Autodesk Inventor part; units mm, degrees
ref_plane "YZ Plane" through (0, 0, 0) normal (1, 0, 0) x (0, 1, 0)
ref_plane "XZ Plane" through (0, 0, 0) normal (0, 1, 0) x (-1, 0, 0)
ref_plane "XY Plane" through (0, 0, 0) normal (0, 0, 1) x (1, 0, 0)
sketch "スケッチ1" plane through (0, 0, 0) normal (1, 0, 0) x (0, 1, 0)
  circle A0 centre (0, 0) radius 4.575
  circle A1 centre (0, 0) radius 3.575
  line L0 (0, 0) -> (0, 6)
  line L1 (0, 6) -> (0, -6)
  line L2 (0, 0) -> (11.5, 0)
  line L3 (11.5, 0) -> (11.5, 9.5)
  line L4 (11.5, 9.5) -> (11.5, -9.5)
  circle A2 centre (11.5, 9.5) radius 1.65
  circle A3 centre (11.5, -9.5) radius 1.65
  line L5 (0, 0) -> (0, 11.25)
  line L6 (0, 11.25) -> (0, -11.25)
  line L7 (-2.5, -11.25) -> (2.5, -11.25)
  line L8 (2.5, -11.25) -> (2.5, 11.25)
  line L9 (2.5, 11.25) -> (-2.5, 11.25)
  line L10 (-2.5, 11.25) -> (-2.5, -11.25)
  line L11 (-2.5, -11.25) -> (2.5, 11.25) construction
  line L12 (2.5, -11.25) -> (-2.5, 11.25) construction
  circle A4 centre (11.5, 9.5) radius 2.5
  circle A5 centre (11.5, -9.5) radius 2.5
  line L13 (2.5, 11.25) -> (11.2899, 11.9912)
  line L14 (2.5, -11.25) -> (11.2899, -11.9912)
  line L15 (14, 9.5) -> (14, -9.5)
  line L16 (0, -3.575) -> (14, -3.575)
  line L17 (0, 3.575) -> (14, 3.575)
  circle A6 centre (0, 0) radius 6
  line L18 (0, 0) -> (0, 6.15)
  line L19 (0, 6.15) -> (0, -6.15)
  circle A7 centre (0, 6.15) radius 1.25
  circle A8 centre (0, -6.15) radius 1.25
  point P0 (0, 4.575)
  point P1 (0, -4.575)
  point P2 (2.5, 3.575)
  point P3 (2.5, 2.5555)
  point P4 (2.5, -2.5555)
  point P5 (2.5, -3.575)
  point P6 (0, 7.4)
  point P7 (0, 4.9)
  point P8 (0, -4.9)
  point P9 (0, -7.4)
  point P10 (2.5, 5.4544)
  point P11 (2.5, -5.4544)
  point P12 (4.8186, 3.575)
  point P13 (4.8186, -3.575)
  point P14 (2.8548, 3.575)
  point P15 (2.8548, -3.575)
  dimension "d0" = 9.15
  dimension "d1" = 7.15
  dimension "d2" = 6
  dimension "d3" = 12
  dimension "d6" = 11.5
  dimension "d7" = 9.5
  dimension "d8" = 19
  dimension "d9" = 3.3
  dimension "d10" = 3.3
  dimension "d11" = 11.25
  dimension "d12" = 22.5
  dimension "d13" = 5
  dimension "d14" = 5
  dimension "d15" = 5
  dimension "d28" = 12
  dimension "d29" = 6.15
  dimension "d30" = 12.3
  dimension "d31" = 2.5
  dimension "d32" = 2.5
extrude "押し出し7" add sketch "スケッチ1" along normal blind 2 contours L2 A6 L16 A0 | A0 L17 A6 L2 | A0 L8 A6 L17 | L16 A6 L8 A0 | A6 L17 L3 L2 | L2 L4 L16 A6 | A0 L0 A7 A6 L8 | A6 L8 L13 A4 L3 L17 | L8 A6 A8 L1 A0 | L16 L4 A5 L14 L8 A6 | L3 L17 L15 L16 L4 | A6 A7 L5 L9 L8 | L3 A4 L15 L17 | L8 L7 L6 A8 A6 | L16 L15 A5 L4 | A4 | A5
extrude "押し出し8" add sketch "スケッチ1" along normal blind 10 contours L2 A6 L16 A0 | A0 L17 A6 L2 | A0 L8 A6 L17 | L16 A6 L8 A0 | A6 L17 L3 L2 | L2 L4 L16 A6 | A0 L0 A7 A6 L8 | L8 A6 A8 L1 A0 | L3 L17 L15 L16 L4 | A6 A7 L5 L9 L8 | L8 L7 L6 A8 A6 | L0 A6 A7 | A6 L5 A7 | A8 A6 L1 | A8 L6 A6 picked at (0.2292, 5.6392) picked at (0.3961, 6.4211) picked at (0.2292, -5.6392) picked at (0.3961, -6.4211)
sketch "スケッチ6" plane through (10, 0, 0) normal (1, 0, 0) x (0, 0, -1)
  line L0 (0, 0) -> (-6.15, 0)
  line L1 (-6.15, 0) -> (6.15, 0)
  circle A0 centre (-6.15, 0) radius 1.25
  circle A1 centre (6.15, 0) radius 1.25
  line L2 (-11.25, 2.5) -> (11.25, 2.5)
  line L3 (11.25, 2.5) -> (11.25, -2.5)
  line L4 (11.25, -2.5) -> (-11.25, -2.5)
  line L5 (-11.25, -2.5) -> (-11.25, 2.5)
  line L6 (-11.25, 2.5) -> (11.25, -2.5) construction
  line L7 (11.25, 2.5) -> (-11.25, -2.5) construction
  line L8 (0, 0) -> (0, 11.5)
  line L9 (0, 11.5) -> (-9.5, 11.5)
  line L10 (-9.5, 11.5) -> (9.5, 11.5)
  circle A2 centre (-9.5, 11.5) radius 1.65
  circle A3 centre (-9.5, 11.5) radius 2.5
  circle A4 centre (9.5, 11.5) radius 1.65
  circle A5 centre (9.5, 11.5) radius 2.5
  circle A6 centre (0, 0) radius 6
  circle A7 centre (0, 0) radius 4.575
  arc A8 (11.9912, 11.2899) -> (9.5, 14) centre (9.5, 11.5) ccw
  line L11 (11.25, 2.5) -> (11.9912, 11.2899)
  line L12 (-11.9912, 11.2899) -> (-11.25, 2.5)
  line L13 (-11.25, 2.5) -> (-11.9912, 11.2899)
  line L14 (9.5, 14) -> (-9.5, 14)
  arc A9 (-9.5, 14) -> (-11.9912, 11.2899) centre (-9.5, 11.5) ccw
  line L15 (-9.5, 14) -> (9.5, 14)
  circle A10 centre (0, 0) radius 3.575
  line L16 (-3.575, 14) -> (-3.575, 4.8186)
  line L17 (3.575, -14) -> (-3.575, -14)
  line L18 (-3.575, -14) -> (-3.575, 14)
  line L19 (-3.575, 14) -> (3.575, 14)
  line L20 (3.575, 14) -> (3.575, -14)
  line L21 (3.575, -14) -> (-3.575, 14) construction
  line L22 (-3.575, -14) -> (3.575, 14) construction
  point P0 (-5.4544, 2.5)
  point P1 (5.4544, 2.5)
  point P2 (7, 11.5)
  point P3 (-7, 11.5)
  point P4 (-3.575, 11.5)
  point P5 (-3.575, 4.8186)
  point P6 (-3.575, 2.5)
  point P7 (-2.5555, 2.5)
  point P8 (2.5555, 2.5)
  point P9 (3.575, 2.5)
  point P10 (3.575, 11.5)
  dimension "d69" = 12
  dimension "d56" = 6.15
  dimension "d57" = 12.3
  dimension "d58" = 2.5
  dimension "d59" = 2.5
  dimension "d62" = 11.5
  dimension "d63" = 9.5
  dimension "d64" = 19
  dimension "d65" = 3.3
  dimension "d66" = 5
  dimension "d67" = 3.3
  dimension "d68" = 5
  dimension "d70" = 9.15
  dimension "d79" = 7.15
extrude "押し出し9" add sketch "スケッチ6" against normal blind 2 contours L2 L12 A3 L9 L16 A6 | L16 L9 L8 A6 | A6 L20 L10 A5 L11 L2 | A6 L8 L10 L20 | L16 L14 L20 L10 L9 | L9 A3 L14 L16 | L20 L14 A5 L10 | A3 | A5
extrude "押し出し10" add sketch "スケッチ1" against normal blind 0.5 contours L2 A6 L16 A0 | A0 L17 A6 L2 | A6 L17 L3 L2 | L2 L4 L16 A6 | L3 L17 L15 L16 L4
sketch "スケッチ7" plane through (-0.5, 0, 0) normal (-1, 0, 0) x (0, 0, 1)
  circle A0 centre (0, 0) radius 3.575
  line L0 (-9.5, 14) -> (9.5, 14)
  line L1 (-3.575, 14) -> (3.575, 14)
  circle A1 centre (0, 0) radius 4.575
  line L2 (-11.25, 0) -> (-11.25, 2.5)
  line L3 (11.25, -2.5) -> (-11.25, -2.5)
  line L4 (-11.25, -2.5) -> (-11.25, 2.5)
  line L5 (-11.25, 2.5) -> (11.25, 2.5)
  line L6 (11.25, 2.5) -> (11.25, -2.5)
  line L7 (11.25, -2.5) -> (-11.25, 2.5) construction
  line L8 (-11.25, -2.5) -> (11.25, 2.5) construction
  line L9 (-3.575, 14) -> (-3.575, 0)
  line L10 (3.575, 14) -> (3.575, 0)
  point P0 (-3.575, 2.5)
  point P1 (-2.5555, 2.5)
  point P2 (2.5555, 2.5)
  point P3 (3.575, 2.5)
  dimension "d75" = 7.15
  dimension "d76" = 5
extrude "押し出し11" add sketch "スケッチ7" along normal blind 3 contours A0 L5 L9 A1 L10 | A1 L9 L0 L10
extrude "押し出し12" add sketch "スケッチ6" along normal blind 3 contours L2 L18 A7 L8 A10 | A10 L8 A7 L20 L2 | L18 A6 L8 A7 | A7 L8 A6 L20 | L16 L9 L8 A6 | A6 L8 L10 L20 | L16 L14 L20 L10 L9
hole "穴1" at (0, 0, -6.15) at (0, 0, 6.15) direction (1, 0, 0) diameter 2.4 depth 3
properties part number "ikafly5.0c"
Verification items for the finished model (mm, model axes). A direction names the side the tool comes from. Coordinates: 2 decimals unless noted, no trailing zeros. Loops run counter-clockwise (first coordinate to the right, second up) from the corner with the lowest first, then second, coordinate; pieces in that order, holes last. Notation, with made-up numbers: (-4, 47.5) -> (7, 47.5) arc R9 cw to (7, 53.5) -> close; hole circle Ø11 at (71, 21.25). An arc over 180 degrees is marked (long way). Answer in a Markdown table with one row per item. Add a question column.
1. Section check D-D, the plane x = 7.25. Enter the section's corners in (y, z) (3 decimals).
2. Section check B-B, the plane y = 4. Enter the section's corners in (x, z) (1 decimal), then the cut area to 3 significant figures.
3. Depth check by flat-ended pin: P1, Ø1.3, axis at y = 0.5, z = -5.5, coming from the -X side; P2, Ø1.5, axis at x = 2.5, z = -1, coming from the -Y side; P3, Ø4, axis at y = 3.5, z = -4.5, coming from the -X side; P4, Ø1.8, axis at x = -2.5, y = 10.5, coming from the -Z side (3 decimals). Enter the tip coordinate at first touch or a pass-through.
4. Section check A-A, the plane z = 9. Enter the section's corners in (x, y), then the cut area to 3 significant figures.
5. Material ranges on probe 1 along Z at (x, y) = (1.3, 11.5); probe 2 along X at (y, z) = (7.75, 6); probe 3 along X at (y, z) = (4.25, -0.5), recorded low to high. Write a range as [from, to].
6. Access from +Z, -Z, +X, -X, +Y, -Y to the whole of each face (thin tool, end or side, straight path). Record for faces 1 (the face through (10, 7, -8)), 2 (the face through (-2, 8, 3.575)), 3 (the face through (5, 9, 3.575)).
7. Section check C-C, the plane z = 6.15. Enter the section's corners in (x, y), then the cut area to 3 significant figures.
8. Draft check along Z on faces 4 (the face through (-1.979, 3.575, -0.04)), 5 (the face through (2, 8, 8)), 6 (the face through (5, 1, 11.25)). Enter one of: +Z half, -Z half, draft (parallel to the pull), parting line (faces both ways), or undercut.
Derived:
| question | item | result |
|---|---|---|
| 1 | outline | (0, -11.25) -> (2.5, -11.25) -> (2.5, -5.454) arc R6 ccw to (4.819, -3.575) -> (14, -3.575) -> (14, 3.575) -> (4.819, 3.575) arc R6 ccw to (2.5, 5.454) -> (2.5, 11.25) -> (0, 11.25) -> (0, 4.575) arc R4.575 cw to (0, -4.575) -> close |
| 2 | outline | (-3.5, -3.6) -> (0, -3.6) -> (0, -11.4) -> (2, -11.4) -> (2, -4.5) -> (8, -4.5) -> (8, -11.4) -> (10, -11.4) -> (10, -3.6) -> (13, -3.6) -> (13, 3.6) -> (10, 3.6) -> (10, 11.4) -> (8, 11.4) -> (8, 4.5) -> (2, 4.5) -> (2, 11.4) -> (0, 11.4) -> (0, 3.6) -> (-3.5, 3.6) -> close; hole (-0.5, -2.2) -> (10, -2.2) -> (10, 2.2) -> (-0.5, 2.2) -> close |
| 2 | area | 145 mm² |
| 3 | P1 | stops at x = 0 |
| 3 | P2 | stops at y = 4.23 |
| 3 | P3 | stops at x = -3.5 |
| 3 | P4 | stops at z = -3.575 |
| 4 | outline | (0, 0) -> (10, 0) -> (10, 9.93) -> (8, 9.93) -> (8, 2.5) -> (2, 2.5) -> (2, 9.93) -> (0, 9.93) -> close; (0, 13.07) -> (2, 13.07) -> (2, 14) -> (0, 14) -> close; (8, 13.07) -> (10, 13.07) -> (10, 14) -> (8, 14) -> close |
| 4 | area | 58.4 mm² |
| 5 | probe 1 | z = [-12, -11.15], [-7.85, 7.85], [11.15, 12] |
| 5 | probe 2 | x = [0, 2], [8, 10] |
| 5 | probe 3 | x = [-3.5, -0.5], [10, 13] |
| 6 | face 1 | -Z, +X, +Y, -Y |
| 6 | face 2 | +Z, -X, +Y, -Y |
| 6 | face 3 | +Z, +Y |
| 7 | outline | (0, 1.2) -> (3, 1.2) -> (3, 0) -> (10, 0) -> (10, 14) -> (8, 14) -> (8, 2.5) -> (2, 2.5) -> (2, 14) -> (0, 14) -> close |
| 7 | area | 67.4 mm² |
| 8 | face 4 | undercut |
| 8 | face 5 | draft |
| 8 | face 6 | +Z half |
